For this review, take the finished solid that the model builds, in its own axes (mm). Face numbers are marked on the shaded views. A direction names the side the tool comes from. Round coordinates to 2 decimals unless told otherwise and drop trailing zeros. Loops run counter-clockwise (first coordinate to the right, second up) from the corner with the lowest first, then second, coordinate; pieces in that order, holes last. Notation, with made-up numbers: (29, 41.25) -> (62, 41.25) arc R28 ccw to (62, 66.25) -> close; hole circle Ø9 at (82, 10). An arc over 180 degrees is marked (long way). Use one line per item in the form item = value. Start each with the question number.
from build123d import *

# Parameters (mm, degrees)
SKETCH_1_R            = 3
EXTRUDE_251_DEPTH     = 2.5
CHAMFER_1_SIZE        = 1.5
CUT_EXTRUDE_459_DEPTH = 1.3
SKETCH_3_R            = 1.5
EXTRUDE_571_DEPTH     = 40


with BuildPart() as part:
    # 草图1 → Extrude 251 (new body)
    with BuildSketch(Plane(origin=(0, 0, 0), x_dir=(1, 0, 0), z_dir=(0, 1, 0))):
        Circle(SKETCH_1_R)
    extrude(amount=EXTRUDE_251_DEPTH)

    # 倒角1
    chamfer_1_edges = [part.edges().sort_by_distance(p)[0] for p in [
        (-3, 0, 0),
    ]]
    chamfer(chamfer_1_edges, length=CHAMFER_1_SIZE)

    # 草图2 → Cut-Extrude 459 (cut)
    with BuildSketch(Plane(origin=(0, 2.5, 0), x_dir=(1, 0, 0), z_dir=(0, 1, 0))):
        Polygon((1.443375673, 0), (0.721687836, 1.25), (-0.721687836, 1.25), (-1.443375673, 0), (-0.721687836, -1.25), (0.721687836, -1.25), align=None)
    extrude(amount=-CUT_EXTRUDE_459_DEPTH, mode=Mode.SUBTRACT)

    # 草图3 → Extrude 571 (add)
    with BuildSketch(Plane.XZ):
        Circle(SKETCH_3_R)
    extrude(amount=EXTRUDE_571_DEPTH)


solid = part.part
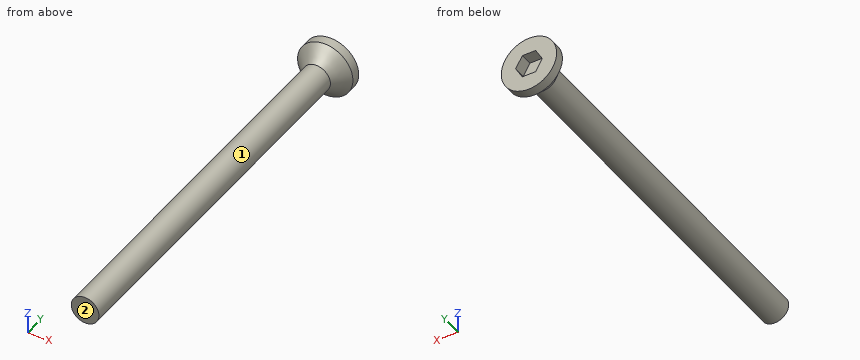
Item 1: Take a section at B-B on y = -26.5. Give the boundary of the cut face in (x, z).
Item 2: Machinability: for the marked faces 1 and 2, which of the approach directions +Z, -Z, +X, -X, +Y, -Y give a long, thin tool a straight path to every point of the face, cutting with its end or side? Answer none if there is none.
Item 3: Wall thickness on line 1 (Y direction, x = -0.5, z = -0.7); line 2 (X direction, y = -31.5, z = 0); line 3 (Z direction, x = -0.4, y = -4): over which ranges is each line inside the solid? List them lowest first.
Item 4: For P1, Ø1.5, axis at x = 2, z = 2.5, coming from the -Y side; P2, Ø2, axis at x = -1, y = -4.5, coming from the +Z side, all flat-tipped, find the tip position at first contact; note any pin that passes through.
Item 5: Take a section at A-A on x = 0. Give the boundary of the cut face in (y, z).
Results:
q1.outline = circle Ø3 at (0, 0)
q2.face_1 = -Y
q2.face_2 = +Z, -Z, +X, -X, -Y
q3.line_1 = -40 to 1.2
q3.line_2 = -1.5 to 1.5
q3.line_3 = -1.45 to 1.45
q4.P1 = 0.95
q4.P2 = 1.5
q5.outline = (-40, -1.5) -> (0, -1.5) -> (1.5, -3) -> (2.5, -3) -> (2.5, -1.25) -> (1.2, -1.25) -> (1.2, 1.25) -> (2.5, 1.25) -> (2.5, 3) -> (1.5, 3) -> (0, 1.5) -> (-40, 1.5) -> close
